from build123d import *

# Parameters (mm, degrees)
SKETCH1_W            = 60
SKETCH1_H            = 30
BOSS_EXTRUDE1_DEPTH  = 10
SKETCH2_W            = 2.7
SKETCH2_H            = 30
BOSS_EXTRUDE2_DEPTH  = 30
CUT_EXTRUDE1_REACH   = 73.472
SKETCH3_R            = 3.23
FILLET1_R            = 3
FILLET1_OF_MIRROR1_R = 3
FILLET4_R            = 2
CUT_EXTRUDE3_REACH   = 73.472
SKETCH5_R            = 1.98
SKETCH5_R_2          = 1.475
CUT_EXTRUDE4_REACH   = 47
SKETCH6_R            = 0.86
FILLET6_R            = 1
SKETCH7_R            = 2.725
SKETCH7_R_2          = 3.23
CUT_EXTRUDE5_DEPTH   = 1.35
SKETCH8_R            = 2
CUT_EXTRUDE6_DEPTH   = 3
CUT_EXTRUDE7_REACH   = 47
SKETCH9_R            = 1


with BuildPart() as part:
    # Sketch1 → Boss-Extrude1 (new body)
    with BuildSketch(Plane(origin=(0, 0, 0), x_dir=(1, 0, 0), z_dir=(0, 1, 0))):
        Rectangle(SKETCH1_W, SKETCH1_H)
    extrude(amount=BOSS_EXTRUDE1_DEPTH)

    # Sketch2 → Boss-Extrude2 (add)
    with BuildSketch(Plane(origin=(0, 10, 0), x_dir=(1, 0, 0), z_dir=(0, 1, 0))):
        with Locations((-28.65, 0)):
            Rectangle(SKETCH2_W, SKETCH2_H)
    boss_extrude2 = extrude(amount=BOSS_EXTRUDE2_DEPTH)

    # Sketch3 → Cut-Extrude1 (cut, up to next)
    with BuildSketch(Plane(origin=(-27.3, 0, 0), x_dir=(0, 0, -1), z_dir=(1, 0, 0)), mode=Mode.PRIVATE) as cut_extrude1_sk1:
        with Locations((0, 36)):
            Circle(SKETCH3_R)
    cut_extrude1_tool1 = extrude(cut_extrude1_sk1.sketch, amount=-CUT_EXTRUDE1_REACH, mode=Mode.PRIVATE) & part.part
    cut_extrude1 = cut_extrude1_tool1.solids().sort_by_distance((-27.3, 36, 0))[0]
    add(cut_extrude1, mode=Mode.SUBTRACT)

    # Fillet1
    fillet1_edges = [part.edges().sort_by_distance(p)[0] for p in [
        (-28.65, 40, 15),
        (-28.65, 40, -15),
    ]]
    fillet(fillet1_edges, radius=FILLET1_R)

    # Mirror1: Boss-Extrude2, Cut-Extrude1 across plane
    add(boss_extrude2.mirror(Plane(origin=(0, 0, 0), x_dir=(0, 0, 1), z_dir=(1, 0, 0))))
    add(cut_extrude1.mirror(Plane(origin=(0, 0, 0), x_dir=(0, 0, 1), z_dir=(1, 0, 0))), mode=Mode.SUBTRACT)

    # Fillet1 of Mirror1
    fillet1_of_mirror1_edges = [part.edges().sort_by_distance(p)[0] for p in [
        (28.65, 40, 15),
        (28.65, 40, -15),
    ]]
    fillet(fillet1_of_mirror1_edges, radius=FILLET1_OF_MIRROR1_R)

    # Fillet4
    fillet4_edges = [part.edges().sort_by_distance(p)[0] for p in [
        (0, 10, 15),
        (0, 10, -15),
    ]]
    fillet(fillet4_edges, radius=FILLET4_R)

    # Sketch5 → Cut-Extrude3 (cut, up to next)
    with BuildSketch(Plane.ZY.offset(-27.3), mode=Mode.PRIVATE) as cut_extrude3_sk1:
        with Locations((10.48, 20.25)):
            Circle(SKETCH5_R)
    cut_extrude3_tool1 = extrude(cut_extrude3_sk1.sketch, amount=-CUT_EXTRUDE3_REACH, mode=Mode.PRIVATE) & part.part
    # Sketch5 → Cut-Extrude3 (cut, up to next)
    with BuildSketch(Plane.ZY.offset(-27.3), mode=Mode.PRIVATE) as cut_extrude3_sk2:
        with Locations((9.52, 36)):
            Circle(SKETCH5_R_2)
    cut_extrude3_tool2 = extrude(cut_extrude3_sk2.sketch, amount=-CUT_EXTRUDE3_REACH, mode=Mode.PRIVATE) & part.part
    cut_extrude3_1 = cut_extrude3_tool1.solids().sort_by_distance((27.3, 20.25, 10.48))[0]
    add(cut_extrude3_1, mode=Mode.SUBTRACT)
    cut_extrude3_2 = cut_extrude3_tool2.solids().sort_by_distance((27.3, 36, 9.52))[0]
    add(cut_extrude3_2, mode=Mode.SUBTRACT)
    cut_extrude3 = cut_extrude3_1 + cut_extrude3_2  # Cut-Extrude3 as one shape, for the pattern or mirror that repeats it

    # Mirror2: Cut-Extrude3 across plane
    add(cut_extrude3.mirror(Plane.XY), mode=Mode.SUBTRACT)

    # Sketch6 → Cut-Extrude4 (cut, up to next)
    with BuildSketch(Plane(origin=(0, 10, 0), x_dir=(1, 0, 0), z_dir=(0, 1, 0)), mode=Mode.PRIVATE) as cut_extrude4_sk1:
        with Locations(Location((-12.53, 4.86, 0), (0, 0, 270))):
            Circle(SKETCH6_R)
    cut_extrude4_tool1 = extrude(cut_extrude4_sk1.sketch, amount=-CUT_EXTRUDE4_REACH, mode=Mode.PRIVATE) & part.part
    # Sketch6 → Cut-Extrude4 (cut, up to next)
    with BuildSketch(Plane(origin=(0, 10, 0), x_dir=(1, 0, 0), z_dir=(0, 1, 0)), mode=Mode.PRIVATE) as cut_extrude4_sk2:
        Polygon((-24.8, -3.5), (-24.8, 3.5), (-10, 3.5), (-10, 10.5), (10, 10.5), (10, 3.5), (24.8, 3.5), (24.8, -3.5), (10, -3.5), (10, -10.5), (-10, -10.5), (-10, -3.5), align=None)
    cut_extrude4_tool2 = extrude(cut_extrude4_sk2.sketch, amount=-CUT_EXTRUDE4_REACH, mode=Mode.PRIVATE) & part.part
    add(cut_extrude4_tool1.solids().sort_by_distance((-12.53, 10, -4.86))[0], mode=Mode.SUBTRACT)
    add(cut_extrude4_tool2.solids().sort_by_distance((0, 10, 0))[0], mode=Mode.SUBTRACT)

    # Fillet6
    fillet6_edges = [part.edges().sort_by_distance(p)[0] for p in [
        (-24.8, 5, -3.5),
        (-10, 5, -3.5),
        (-10, 5, -10.5),
        (10, 5, -10.5),
        (10, 5, -3.5),
        (24.8, 5, -3.5),
        (24.8, 5, 3.5),
        (10, 5, 3.5),
        (10, 5, 10.5),
        (-10, 5, 10.5),
        (-10, 5, 3.5),
        (-24.8, 5, 3.5),
    ]]
    fillet(fillet6_edges, radius=FILLET6_R)

    # Sketch7 → Cut-Extrude5 (cut)
    with BuildSketch(Plane.ZY.offset(-27.3)):
        with Locations((-9.52, 36)):
            Circle(SKETCH7_R)
        with Locations((-10.48, 20.25)):
            Circle(SKETCH7_R_2)
        with Locations((10.48, 20.25)):
            Circle(SKETCH7_R_2)
        with Locations((9.52, 36)):
            Circle(SKETCH7_R)
    extrude(amount=-CUT_EXTRUDE5_DEPTH, mode=Mode.SUBTRACT)

    # Sketch8 → Cut-Extrude6 (cut)
    with BuildSketch(Plane(origin=(0, 10, 0), x_dir=(1, 0, 0), z_dir=(0, 1, 0))):
        with Locations(Location((-23.3, 10, 0), (0, 0, 270))):
            Circle(SKETCH8_R)
        with Locations(Location((-23.3, -10, 0), (0, 0, 270))):
            Circle(SKETCH8_R)
    cut_extrude6 = extrude(amount=-CUT_EXTRUDE6_DEPTH, mode=Mode.SUBTRACT)

    # Sketch9 → Cut-Extrude7 (cut, up to next)
    with BuildSketch(Plane(origin=(0, 10, 0), x_dir=(1, 0, 0), z_dir=(0, 1, 0)), mode=Mode.PRIVATE) as cut_extrude7_sk1:
        with Locations(Location((-23.3, 10, 0), (0, 0, 270))):
            Circle(SKETCH9_R)
    cut_extrude7_tool1 = extrude(cut_extrude7_sk1.sketch, amount=-CUT_EXTRUDE7_REACH, mode=Mode.PRIVATE) & part.part
    # Sketch9 → Cut-Extrude7 (cut, up to next)
    with BuildSketch(Plane(origin=(0, 10, 0), x_dir=(1, 0, 0), z_dir=(0, 1, 0)), mode=Mode.PRIVATE) as cut_extrude7_sk2:
        with Locations(Location((-23.3, -10, 0), (0, 0, 270))):
            Circle(SKETCH9_R)
    cut_extrude7_tool2 = extrude(cut_extrude7_sk2.sketch, amount=-CUT_EXTRUDE7_REACH, mode=Mode.PRIVATE) & part.part
    cut_extrude7_1 = cut_extrude7_tool1.solids().sort_by_distance((-23.3, 10, -10))[0]
    add(cut_extrude7_1, mode=Mode.SUBTRACT)
    cut_extrude7_2 = cut_extrude7_tool2.solids().sort_by_distance((-23.3, 10, 10))[0]
    add(cut_extrude7_2, mode=Mode.SUBTRACT)
    cut_extrude7 = cut_extrude7_1 + cut_extrude7_2  # Cut-Extrude7 as one shape, for the pattern or mirror that repeats it

    # Mirror3: Cut-Extrude6, Cut-Extrude7 across plane
    add(cut_extrude6.mirror(Plane(origin=(0, 0, 0), x_dir=(0, 0, 1), z_dir=(1, 0, 0))), mode=Mode.SUBTRACT)
    add(cut_extrude7.mirror(Plane(origin=(0, 0, 0), x_dir=(0, 0, 1), z_dir=(1, 0, 0))), mode=Mode.SUBTRACT)


solid = part.part
The listing builds one solid part. Answer for the finished solid, in the listing's coordinates (mm). A direction names the side the tool comes from. Give positions to 0.01 mm unless a question says otherwise; leave off trailing zeros. Write each loop counter-clockwise with the first axis right and the second up, starting at its lowest first coordinate (ties: lowest second). Pieces come first, ordered by that corner, then holes.
Item 1: Section A-A, the plane z = 0 is taken. Write down the section's boundary in (x, y), plus the area to 3 significant figures.
Item 2: Which of the six approach directions +Z, -Z, +X, -X, +Y, -Y give full straight-line access (tool end or side, diameter ignored) to faces 5 (the flat face through (0, 5, 10.5)), 6 (the cylindrical face through (0.38, 9.4, -14.43)), 7 (the cylindrical face through (28.631, 32.847, 0.7)), 8 (the cylindrical face through (27.966, 17.097, 9.78))?
Item 3: Flat-ended cylindrical pins translate along their axes: P1, Ø2, axis at x = -23, z = -10, coming from the +Y side; P2, Ø8, axis at x = -17, z = -9, coming from the +Y side; P3, Ø12, axis at x = -1.5, y = 17, coming from the +Z side. Find the tip coordinate at first contact, or state that the pin passes through.
Item 4: Section C-C, the plane y = 28 is taken. Write down the section's boundary in (x, z), plus the area to 3 significant figures.
Item 5: Section D-D, the plane x = -12.53 is taken. Write down the section's boundary in (y, z).
Item 6: Find the intervals of material crossed by line 1 along X through (y, z) = (3, -4.86); line 2 along X through (y, z) = (37.5, 7); line 3 along X through (y, z) = (4.5, 10), in increasing order.
Item 7: Section B-B, the plane x = 14.5 is taken. Write down the section's boundary in (y, z), plus the area to 3 significant figures.
Item 8: Determine the mould class of faces 1 (the flat face through (30, 20, 0)), 2 (the flat face through (-22, 7, 10)), 3 (the cylindrical face through (-25.252, 8.521, 9.566)), 4 (the flat face through (0, 0, -14)) for opening direction X: released by +X, released by -X, zero draft, split by the parting line, or undercut.
Completed:
1. outline: (-30, 0) - (-24.8, 0) - (-24.8, 10) - (-27.3, 10) - (-27.3, 32.77) - (-30, 32.77) - close; (-30, 39.23) - (-27.3, 39.23) - (-27.3, 40) - (-30, 40) - close; (24.8, 0) - (30, 0) - (30, 32.77) - (27.3, 32.77) - (27.3, 10) - (24.8, 10) - close; (27.3, 39.23) - (30, 39.23) - (30, 40) - (27.3, 40) - close
1. area: 231 mm2
2. face 5: +Y, -Y
2. face 6: -Z, +Y
2. face 7: +X, -X
2. face 8: none
3. P1: stops at y = 7
3. P2: stops at y = 10
3. P3: passes through
4. outline: (-30, -15) - (-27.3, -15) - (-27.3, 15) - (-30, 15) - close; (27.3, -15) - (30, -15) - (30, 15) - (27.3, 15) - close
4. area: 162 mm2
5. outline: (0, -15) - (8, -15) arc R2 ccw to (10, -13) - (10, -5.72) - (0, -5.72) - close; (0, -4) - (10, -4) - (10, -3.5) - (0, -3.5) - close; (0, 3.5) - (10, 3.5) - (10, 13) arc R2 ccw to (8, 15) - (0, 15) - close
6. line 1: x = -30 to -13.39, -11.67 to -10, 10 to 30
6. line 2: x = -30 to -27.3, 27.3 to 30
6. line 3: x = -30 to -24.3, -22.3 to -9.87, 9.87 to 22.3, 24.3 to 30
7. outline: (0, -15) - (8, -15) arc R2 ccw to (10, -13) - (10, -3.5) - (0, -3.5) - close; (0, 3.5) - (10, 3.5) - (10, 13) arc R2 ccw to (8, 15) - (0, 15) - close
7. area: 228 mm2
8. face 1: released by +X
8. face 2: undercut
8. face 3: undercut
8. face 4: zero draft
